Can you work these out from the model? Positions are in its coordinate system, mm. A direction names the side the tool comes from. Coordinates: 2 decimals unless noted, no trailing zeros. Order: outer loops, then holes, each group sorted by start corner. A loop starts at its lowest first (then second) coordinate and runs counter-clockwise, first axis right, second up. Notation, with made-up numbers: M 36.5,-3 L 80.5,-3 A28 cw 80.5,15 Z; hole C -12.75,60 d3. An arc over 180 degrees is marked long. Answer as CSV lines item,"result". Start each with the question number.
1. I need wall thicknesses on line 1 along X through (y, z) = (0.75, 0); line 2 along X through (y, z) = (10.9, 0); line 3 along Z through (x, y) = (11.5, -8.75) (3 decimals). Which ranges of each line are inside material? Lowest first, please. Write a range as from..to.
2. If we mould it in two halves opening along Z, with no side actions, what happens to faces 3 (the face through (15.77, 0.175, 50.076)), 4 (the face through (24, -12.5, 39)), 5 (the face through (-17.235, -7.57, -41.569))? For each: released by +Z, released by -Z, zero draft, split by the parting line, or undercut.
3. If we section it at A-A (x = 0): List the corners of the cut face in (y, z) for me.
4. If we section it at C-C (y = 3.25): List the corners of the cut face in (x, z) for me, plus the area to 3 significant figures.
5. Will these pins go through, and if not, where does the flat tip stop? pin 1 (1 mm diameter, centred on x = -23.5, y = -2.5, fed in from -Z); pin 2 (1.5 mm diameter, centred on x = 20, y = -6, fed in from +Z); pin 3 (5 mm diameter, centred on x = -29, y = -2.5, fed in from +Z).
6. If we section it at B-B (z = 0): List the corners of the cut face in (x, y) for me.
7. If we section it at D-D (z = -40): List the corners of the cut face in (x, y) for me, plus the area to 3 significant figures.
8. On a 3-axis mill with a long thin cutter (end or side, diameter ignored), from which of +Z, -Z, +X, -X, +Y, -Y can I reach the whole of each face in a straight line? I mean faces 1 (the face through (26.274, 9.458, 3.45)), 2 (the face through (-33.12, -2.5, 10.21)). Say none if no direction works.
```python
from build123d import *

# Parameters (mm, degrees)
SKETCH1_R           = 52.5
BOSS_EXTRUDE1_DEPTH = 12.5
SKETCH3_R           = 45
CUT_EXTRUDE1_DEPTH  = 10
SKETCH4_R           = 34.5
CUT_EXTRUDE2_DEPTH  = 9
SKETCH5_R           = 26.5
CUT_EXTRUDE3_DEPTH  = 22


with BuildPart() as part:
    # Sketch1 → Boss-Extrude1 (new, symmetric)
    with BuildSketch(Plane(origin=(0, 0, 0), x_dir=(-1, 0, 0), z_dir=(0, 1, 0))):
        with Locations(Location((0, 0, 0), (0, 0, 90))):
            Circle(SKETCH1_R)
    extrude(amount=BOSS_EXTRUDE1_DEPTH, both=True)

    # Sketch3 → Cut-Extrude1 (cut)
    with BuildSketch(Plane.XZ.offset(12.5)):
        with Locations(Location((0, 0, 0), (0, 0, 270))):
            Circle(SKETCH3_R)
    extrude(amount=-CUT_EXTRUDE1_DEPTH, mode=Mode.SUBTRACT)

    # Sketch4 → Cut-Extrude2 (cut)
    with BuildSketch(Plane.XZ.offset(2.5)):
        with Locations(Location((0, 0, 0), (0, 0, 270))):
            Circle(SKETCH4_R)
    extrude(amount=-CUT_EXTRUDE2_DEPTH, mode=Mode.SUBTRACT)

    # Sketch5 → Cut-Extrude3 (cut)
    with BuildSketch(Plane.XZ.offset(-6.5)):
        with Locations(Location((0, 0, 0), (0, 0, 270))):
            Circle(SKETCH5_R)
    extrude(amount=-CUT_EXTRUDE3_DEPTH, mode=Mode.SUBTRACT)


solid = part.part
```
Solved:
1,line 1,"-52.5..-34.5, 34.5..52.5"
1,line 2,"-52.5..-26.5, 26.5..52.5"
1,line 3,"-51.225..-43.506, 43.506..51.225"
2,face 3,"split by the parting line"
2,face 4,"zero draft"
2,face 5,"undercut"
3,outline,"M -12.5,-52.5 L 12.5,-52.5 L 12.5,-26.5 L 6.5,-26.5 L 6.5,-34.5 L -2.5,-34.5 L -2.5,-45 L -12.5,-45 Z; M -12.5,45 L -2.5,45 L -2.5,34.5 L 6.5,34.5 L 6.5,26.5 L 12.5,26.5 L 12.5,52.5 L -12.5,52.5 Z"
4,outline,"C 0,0 d105; hole C 0,0 d69"
4,area,"4,920 mm²"
5,pin 1,"z = -47.19"
5,pin 2,"z = 48.84"
5,pin 3,"z = 45.32"
6,outline,"M -52.5,-12.5 L -45,-12.5 L -45,-2.5 L -34.5,-2.5 L -34.5,6.5 L -26.5,6.5 L -26.5,12.5 L -52.5,12.5 Z; M 26.5,6.5 L 34.5,6.5 L 34.5,-2.5 L 45,-2.5 L 45,-12.5 L 52.5,-12.5 L 52.5,12.5 L 26.5,12.5 Z"
7,outline,"M -34,-12.5 L -20.62,-12.5 L -20.62,-2.5 L 20.62,-2.5 L 20.62,-12.5 L 34,-12.5 L 34,12.5 L -34,12.5 Z"
7,area,"1,290 mm²"
8,face 1,"+Y, -Y"
8,face 2,"-Y"
